from build123d import *

# Parameters (mm, degrees)
SKETCH1_W                = 15
SKETCH1_H                = 50
BOSS_EXTRUDE1_DEPTH      = 1.6
M12_MOUNTING_HOLES_REACH = 31.199
SKETCH3_R                = 0.6
SKETCH3_R_2              = 0.65


with BuildPart() as part:
    # Sketch1 → Boss-Extrude1 (new body)
    with BuildSketch(Plane(origin=(0, 0, 0), x_dir=(1, 0, 0), z_dir=(0, 1, 0))):
        with Locations((7.5, 0)):
            Rectangle(SKETCH1_W, SKETCH1_H)
    extrude(amount=BOSS_EXTRUDE1_DEPTH)

    # Sketch3 → M12 mounting holes (cut, up to next)
    with BuildSketch(Plane(origin=(0, 1.6, 0), x_dir=(1, 0, 0), z_dir=(0, 1, 0)), mode=Mode.PRIVATE) as m12_mounting_holes_sk1:
        with Locations(Location((5, 0, 0), (0, 0, 270))):
            Circle(SKETCH3_R)
    m12_mounting_holes_tool1 = extrude(m12_mounting_holes_sk1.sketch, amount=-M12_MOUNTING_HOLES_REACH, mode=Mode.PRIVATE) & part.part
    # Sketch3 → M12 mounting holes (cut, up to next)
    with BuildSketch(Plane(origin=(0, 1.6, 0), x_dir=(1, 0, 0), z_dir=(0, 1, 0)), mode=Mode.PRIVATE) as m12_mounting_holes_sk2:
        with Locations(Location((3.232233047, 1.767766953, 0), (0, 0, 270))):
            Circle(SKETCH3_R)
    m12_mounting_holes_tool2 = extrude(m12_mounting_holes_sk2.sketch, amount=-M12_MOUNTING_HOLES_REACH, mode=Mode.PRIVATE) & part.part
    # Sketch3 → M12 mounting holes (cut, up to next)
    with BuildSketch(Plane(origin=(0, 1.6, 0), x_dir=(1, 0, 0), z_dir=(0, 1, 0)), mode=Mode.PRIVATE) as m12_mounting_holes_sk3:
        with Locations(Location((6.767766953, 1.767766953, 0), (0, 0, 270))):
            Circle(SKETCH3_R)
    m12_mounting_holes_tool3 = extrude(m12_mounting_holes_sk3.sketch, amount=-M12_MOUNTING_HOLES_REACH, mode=Mode.PRIVATE) & part.part
    # Sketch3 → M12 mounting holes (cut, up to next)
    with BuildSketch(Plane(origin=(0, 1.6, 0), x_dir=(1, 0, 0), z_dir=(0, 1, 0)), mode=Mode.PRIVATE) as m12_mounting_holes_sk4:
        with Locations(Location((6.767766953, -1.767766953, 0), (0, 0, 270))):
            Circle(SKETCH3_R)
    m12_mounting_holes_tool4 = extrude(m12_mounting_holes_sk4.sketch, amount=-M12_MOUNTING_HOLES_REACH, mode=Mode.PRIVATE) & part.part
    # Sketch3 → M12 mounting holes (cut, up to next)
    with BuildSketch(Plane(origin=(0, 1.6, 0), x_dir=(1, 0, 0), z_dir=(0, 1, 0)), mode=Mode.PRIVATE) as m12_mounting_holes_sk5:
        with Locations(Location((3.232233047, -1.767766953, 0), (0, 0, 270))):
            Circle(SKETCH3_R)
    m12_mounting_holes_tool5 = extrude(m12_mounting_holes_sk5.sketch, amount=-M12_MOUNTING_HOLES_REACH, mode=Mode.PRIVATE) & part.part
    # Sketch3 → M12 mounting holes (cut, up to next)
    with BuildSketch(Plane(origin=(0, 1.6, 0), x_dir=(1, 0, 0), z_dir=(0, 1, 0)), mode=Mode.PRIVATE) as m12_mounting_holes_sk6:
        with Locations(Location((9, 0, 0), (0, 0, 270))):
            Circle(SKETCH3_R_2)
    m12_mounting_holes_tool6 = extrude(m12_mounting_holes_sk6.sketch, amount=-M12_MOUNTING_HOLES_REACH, mode=Mode.PRIVATE) & part.part
    add(m12_mounting_holes_tool1.solids().sort_by_distance((5, 1.6, 0))[0], mode=Mode.SUBTRACT)
    add(m12_mounting_holes_tool2.solids().sort_by_distance((3.232233, 1.6, -1.767767))[0], mode=Mode.SUBTRACT)
    add(m12_mounting_holes_tool3.solids().sort_by_distance((6.767767, 1.6, -1.767767))[0], mode=Mode.SUBTRACT)
    add(m12_mounting_holes_tool4.solids().sort_by_distance((6.767767, 1.6, 1.767767))[0], mode=Mode.SUBTRACT)
    add(m12_mounting_holes_tool5.solids().sort_by_distance((3.232233, 1.6, 1.767767))[0], mode=Mode.SUBTRACT)
    add(m12_mounting_holes_tool6.solids().sort_by_distance((9, 1.6, 0))[0], mode=Mode.SUBTRACT)


solid = part.part
Source: CAD feature listing. Evaluate the final solid. Frame: model axes, mm. Coordinates: 2 decimals unless noted, no trailing zeros. Loops run counter-clockwise (first coordinate to the right, second up) from the corner with the lowest first, then second, coordinate; pieces in that order, holes last. Notation, with made-up numbers: (30.25, -2.75) -> (41.25, -2.75) arc R11 cw to (41.25, 15.25) -> close; hole circle Ø8 at (74, 82). An arc over 180 degrees is marked (long way). Answer in a Markdown table with one row per item. Add a question column.
Q1. Section C-C on x = 9. Return the cut outline in (y, z), and give its area (3 significant figures).
Q2. Contact query for a flat-ended pin moving along its axis: pin 1 Ø1.4 at (x, z) = (6.77, 1.77) entering from -Y. Output: stop coordinate, or through.
Q3. Ray query, line 1 along X through (y, z) = (1.35, 0); line 2 along Z through (x, y) = (6.75, 0.8); line 3 along Z through (x, y) = (9.25, 1.3). Return the intervals inside material, ascending.
Q4. Section B-B on z = 0. Return the cut outline in (x, y).
Q5. Section A-A on x = 5. Return the cut outline in (y, z), and give its area (3 significant figures).
Computed values:
| question | item | result |
|---|---|---|
| 1 | outline | (0, -25) -> (1.6, -25) -> (1.6, -0.65) -> (0, -0.65) -> close; (0, 0.65) -> (1.6, 0.65) -> (1.6, 25) -> (0, 25) -> close |
| 1 | area | 77.9 mm^2 |
| 2 | pin 1 | stops at y = 0 |
| 3 | line 1 | x = 0 to 4.4, 5.6 to 8.35, 9.65 to 15 |
| 3 | line 2 | z = -25 to -2.37, -1.17 to 1.17, 2.37 to 25 |
| 3 | line 3 | z = -25 to -0.6, 0.6 to 25 |
| 4 | outline | (0, 0) -> (4.4, 0) -> (4.4, 1.6) -> (0, 1.6) -> close; (5.6, 0) -> (8.35, 0) -> (8.35, 1.6) -> (5.6, 1.6) -> close; (9.65, 0) -> (15, 0) -> (15, 1.6) -> (9.65, 1.6) -> close |
| 5 | outline | (0, -25) -> (1.6, -25) -> (1.6, -0.6) -> (0, -0.6) -> close; (0, 0.6) -> (1.6, 0.6) -> (1.6, 25) -> (0, 25) -> close |
| 5 | area | 78.1 mm^2 |
